Can you work these out from the model? Positions are in its coordinate system, mm. Face numbers are marked on the shaded views. A direction names the side the tool comes from. Give positions to 0.01 mm unless a question says otherwise; leave off trailing zeros. Loops run counter-clockwise (first coordinate to the right, second up) from the corner with the lowest first, then second, coordinate; pieces in that order, holes last. Notation, with made-up numbers: M 82,35.25 L 87,35.25 A23 ccw 87,54.25 Z; hole C 9.5,67 d4. An arc over 180 degrees is marked long. Answer as a JSON object with one key per item and string values.
```python
from build123d import *

# Parameters (mm, degrees)
CHAFL_N1_SIZE         = 2
CHAFL_N1_SIZE2        = 0.688655227
CHAFL_N2_SIZE         = 0.5
CROQUIS2_OUTSIDE_W    = 14.998
CROQUIS2_OUTSIDE_H    = 14.998
CROQUIS2_OUTSIDE_W_2  = 8
CROQUIS2_OUTSIDE_H_2  = 12
CORTAR_EXTRUIR1_DEPTH = 4


with BuildPart() as part:
    # Croquis1 → Revolución2 (revolve)
    with BuildSketch(Plane.XY):
        Polygon((2.3, 0), (4.76, 0), (4.76, 5), (4, 5), (4, 11), (3, 11), (3, 1), (1.5, 1), (1.5, 0.8), align=None)
    revolve(axis=Axis((0, 26.23655914, 0), (0, -1, 0)))

    # Chaflán1
    chafl_n1_edges = [part.edges().sort_by_distance(p)[0] for p in [
        (-4.76, 0, 0),
    ]]
    chafl_n1_side = [part.faces().sort_by_distance(p)[0] for p in [
        (-2.434633131, 0, 0),
    ]]
    chamfer(chafl_n1_edges, length=CHAFL_N1_SIZE, length2=CHAFL_N1_SIZE2, reference=chafl_n1_side[0])

    # Chaflán2
    chafl_n2_edges = [part.edges().sort_by_distance(p)[0] for p in [
        (-3, 11, 0),
    ]]
    chamfer(chafl_n2_edges, length=CHAFL_N2_SIZE)

    # Croquis2 outside → Cortar-Extruir1 (cut)
    with BuildSketch(Plane.XZ):
        Rectangle(CROQUIS2_OUTSIDE_W, CROQUIS2_OUTSIDE_H)
        Rectangle(CROQUIS2_OUTSIDE_W_2, CROQUIS2_OUTSIDE_H_2, mode=Mode.SUBTRACT)
    extrude(amount=-CORTAR_EXTRUIR1_DEPTH, mode=Mode.SUBTRACT)


solid = part.part
```
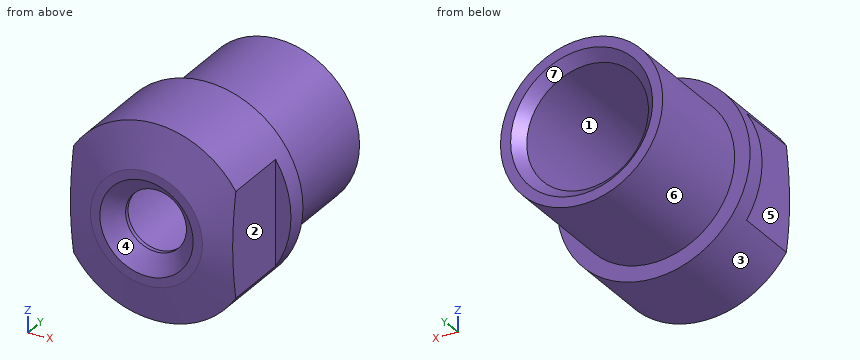
1) If we mould it in two halves opening along Z, with no side actions, what happens to the marked faces 4, 5, 6 and 7? For each: +Z half, -Z half, draft (parallel to the pull), parting line (faces both ways), or undercut.
Answer list:
{"face 4": "undercut", "face 5": "draft", "face 6": "parting line", "face 7": "undercut"}
2) Suppose I cut it at C-C, the plane y = 2.25. Write out the boundary of the cut face in (x, z).
Answer list:
{"outline": "M -4,-2.58 A4.76 ccw 4,-2.58 L 4,2.58 A4.76 ccw -4,2.58 Z; hole C 0,0 d6"}
3) Please list where these lines run through material, in increasing order: line 1 along Z through (x, y) = (0, 4.5); line 2 along Z through (x, y) = (0, 0.9); line 3 along X through (y, z) = (6, 1.75). Write a range as from..to.
Answer list:
{"line 1": "-4.76..-3, 3..4.76", "line 2": "-4.76..-1.5, 1.5..4.76", "line 3": "-3.6..-2.44, 2.44..3.6"}
4) Suppose I cut it at D-D, the plane y = 4.5. Write out the boundary of the cut face in (x, z).
Answer list:
{"outline": "C 0,0 d9.52; hole C 0,0 d6"}
5) Will these pins go through, and if not, where does the flat tip stop? pin 1 Ø1 at (y, z) = (9, -3.5) entering from +X; pin 2 Ø5 at (x, z) = (0, 0) entering from +Y; pin 3 Ø5 at (x, z) = (-0.5, -0.5) entering from +Y.
Answer list:
{"pin 1": "x = 2.65", "pin 2": "y = 1", "pin 3": "y = 10.71"}
6) Suppose I cut it at A-A, the plane z = 0. Write out the boundary of the cut face in (x, y).
Answer list:
{"outline": "M -4.76,4 L -4,4 L -4,0.43 L -2.76,0 L -2.3,0 L -1.5,0.8 L -1.5,1 L -3,1 L -3,10.5 L -3.5,11 L -4,11 L -4,5 L -4.76,5 Z; M 1.5,0.8 L 2.3,0 L 2.76,0 L 4,0.43 L 4,4 L 4.76,4 L 4.76,5 L 4,5 L 4,11 L 3.5,11 L 3,10.5 L 3,1 L 1.5,1 Z"}
7) Suppose I cut it at B-B, the plane x = 0. Write out the boundary of the cut face in (y, z).
Answer list:
{"outline": "M 0,-2.76 L 0.69,-4.76 L 5,-4.76 L 5,-4 L 11,-4 L 11,-3.5 L 10.5,-3 L 1,-3 L 1,-1.5 L 0.8,-1.5 L 0,-2.3 Z; M 0,2.3 L 0.8,1.5 L 1,1.5 L 1,3 L 10.5,3 L 11,3.5 L 11,4 L 5,4 L 5,4.76 L 0.69,4.76 L 0,2.76 Z"}
8) For the marked faces 1, 2 and 3, which set-ups out of +Z, -Z, +X, -X, +Y, -Y let a thin tool reach every point of the face, with its end or its side?
Answer list:
{"face 1": "+Y", "face 2": "+Z, -Z, +X, -Y", "face 3": "+Y, -Y"}
